```python
from build123d import *

# Parameters (mm, degrees)
F1_DEPTH = 4
F2_W     = 39.990724
F2_H     = 8
F2_W_2   = 40.150487
F3_DEPTH = 4
F4_DEPTH = 4
F5_R     = 1.5
F6_DEPTH = 43


with BuildPart() as f1:
    # F0 (on Top) → F1 (new body)
    with BuildSketch(Plane.XY):
        Polygon((-123.954707, -15), (123.954707, -15), (123.954707, -7), (-36.045293, -7), (-36.045293, -4), (84.019206, -4), (84.019206, 4), (83.963744, 4), (83.954707, 4), (-36.045293, 4), (-36.045293, 7), (123.954707, 7), (123.954707, 15), (-123.954707, 15), align=None)
    extrude(amount=F1_DEPTH)

    # F2 (on face) → F3 (join)
    with BuildSketch(Plane.XY.offset(4)):
        with Locations((103.959345, 11)):
            Rectangle(F2_W, F2_H)
        with Locations((103.879463, -11)):
            Rectangle(F2_W_2, F2_H)
    extrude(amount=F3_DEPTH)

    # F2 (on face) → F4 (join)
    with BuildSketch(Plane.XY.offset(4)):
        with Locations((103.959345, 11)):
            Rectangle(F2_W, F2_H)
        with Locations((103.879463, -11)):
            Rectangle(F2_W_2, F2_H)
    extrude(amount=F4_DEPTH)

    # F5 (on face) → F6 (cut)
    with BuildSketch(Plane.XZ.offset(15)):
        with Locations((108.954707, 4)):
            Circle(F5_R)
    extrude(amount=-F6_DEPTH, mode=Mode.SUBTRACT)


solid = f1.part
```
Build history of the part. All positions in model axes, mm. A direction names the side the tool comes from. Give positions to 0.01 mm unless a question says otherwise; leave off trailing zeros. Loops run counter-clockwise (first coordinate to the right, second up) from the corner with the lowest first, then second, coordinate; pieces in that order, holes last.
1) Probe line 1 along Y through (x, z) = (30, 1); line 2 along Y through (x, z) = (94.5, 1.75); line 3 along Z through (x, y) = (-103, -4.5). List the from-to ranges inside material, lowest first.
Values follow:
line 1: y = -15 to -7, -4 to 4, 7 to 15
line 2: y = -15 to -7, 7 to 15
line 3: z = 0 to 4
2) Drop flat-ended pins along their axis: P1, Ø6, axis at x = 77, y = 4, coming from the -Z side; P2, Ø2, axis at y = 10, z = 6.5, coming from the -X side; P3, Ø1.2, axis at y = -9.5, z = 6, coming from the -X side; P4, Ø15, axis at x = -43, y = -3, coming from the +Z side. Give the stop position or say it passes through.
Values follow:
P1: stops at z = 0
P2: stops at x = 83.96
P3: stops at x = 83.8
P4: stops at z = 4
3) Two-plate mould, pull along Y, no slides. Class faces 5 (the face through (123.955, -11, 6)), 6 (the face through (-2, 15, 2)), 7 (the face through (-2, -15, 2)), 8 (the face through (84.019, 0, 2)): released by +Y, released by -Y, zero draft, split by the parting line, or undercut.
Values follow:
face 5: zero draft
face 6: released by +Y
face 7: released by -Y
face 8: undercut
4) 3-axis set-ups, long thin cutter, end or side, ignore diameter. For faces 1 (the face through (83.964, 11, 6)), 2 (the face through (-21, 0, 4)), 3 (the face through (104, -11, 8)), 4 (the face through (23, -4, 2)): which of +Z, -Z, +X, -X, +Y, -Y reach the whole face in a straight line?
Values follow:
face 1: +Z, -X, +Y
face 2: +Z, -X, +Y, -Y
face 3: +Z, +X, -X, +Y, -Y
face 4: +Z, -Z, +X
5) Band-saw the part on B-B on y = 12.5. List the corners of the cut face in (x, z), then the cut area to 3 significant figures.
Values follow:
outline: (-123.95, 0) - (123.95, 0) - (123.95, 8) - (83.96, 8) - (83.96, 4) - (-123.95, 4) - close; hole circle Ø3 at (108.95, 4)
area: 1,140 mm2
6) Band-saw the part on C-C on y = -9.25. List the corners of the cut face in (x, z), then the cut area to 3 significant figures.
Values follow:
outline: (-123.95, 0) - (123.95, 0) - (123.95, 8) - (83.8, 8) - (83.8, 4) - (-123.95, 4) - close; hole circle Ø3 at (108.95, 4)
area: 1,150 mm2
7) Band-saw the part on A-A on x = 44. List the corners of the cut face in (y, z).
Values follow:
outline: (-15, 0) - (-7, 0) - (-7, 4) - (-15, 4) - close; (-4, 0) - (4, 0) - (4, 4) - (-4, 4) - close; (7, 0) - (15, 0) - (15, 4) - (7, 4) - close
